Here's the drawing with two shaded views (mm, measured from the low corner). I have some questions. A direction names the side the tool comes from. Round coordinates to 2 decimals unless told otherwise and drop trailing zeros. Loops run counter-clockwise (first coordinate to the right, second up) from the corner with the lowest first, then second, coordinate; pieces in that order, holes last.
(1) Will these pins go through, and if not, where does the flat tip stop? pin 1 Ø5 at (x, y) = (19, 118) entering from -Z; pin 2 Ø10 at (x, z) = (13.5, 18.5) entering from -Y.
(2) Thinking about a two-plate mould opening in Z: for the marked faces 1, 2 and 3, which applies, released by +Z, released by -Z, zero draft, split by the parting line, or undercut?
(3) I want a section at B-B on y = 37. Write out the boundary of the cut face in (x, z).
(4) I want a section at C-C on x = 9. Write out the boundary of the cut face in (y, z) (1 decimal).
(5) I want a section at A-A on z = 20.25. Write out the boundary of the cut face in (x, y) (1 decimal), plus the area to 3 significant figures.
(6) If I drill on line 1 along X through (y, z) = (228, 19); line 2 along Z through (x, y) = (27.5, 200), over which ranges is the centre line in solid material (lowest first)?
(7) Which directions (+Z, -Z, +X, -X, +Y, -Y) give clear straight access to the entire face, cutting with the end or side of a thin tool? Please do the marked faces 4 and 5.
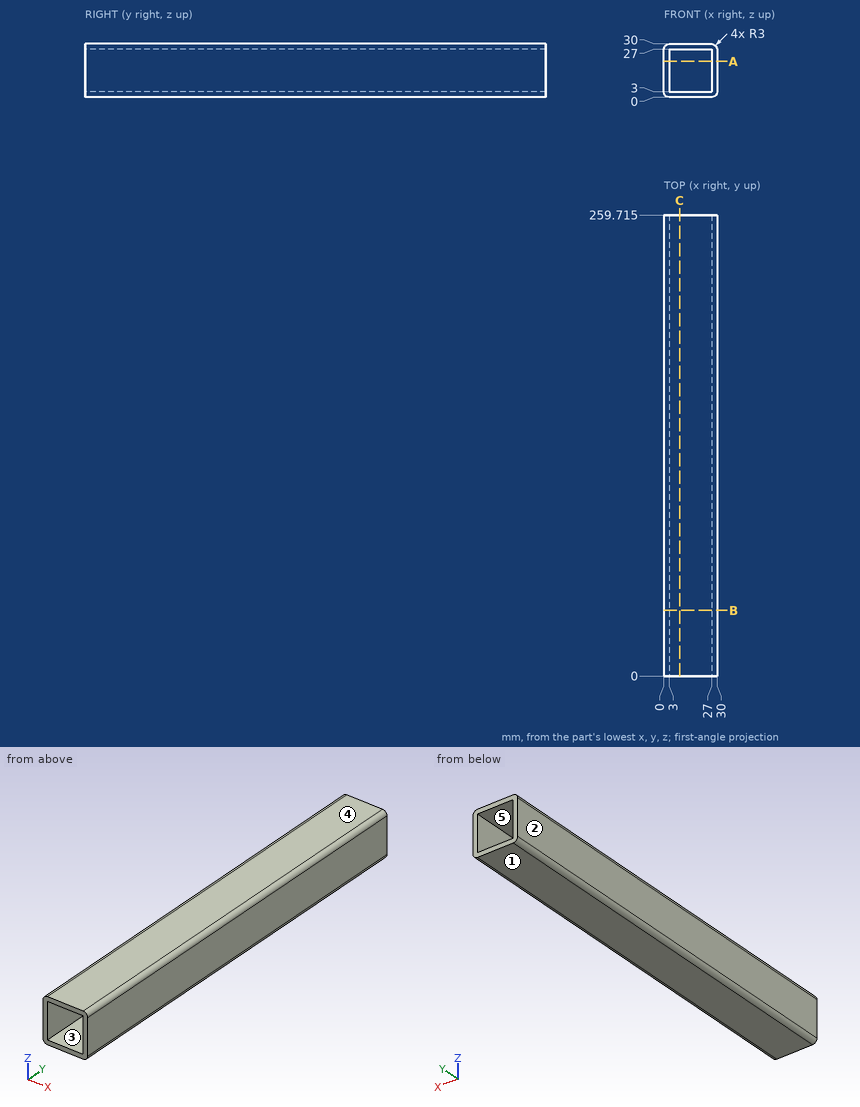
Filled sheet:
1. pin 1: stops at z = 0
1. pin 2: passes through
2. face 1: released by -Z
2. face 2: zero draft
2. face 3: undercut
3. outline: (0, 3) arc R3 ccw to (3, 0) - (27, 0) arc R3 ccw to (30, 3) - (30, 27) arc R3 ccw to (27, 30) - (3, 30) arc R3 ccw to (0, 27) - close; hole (3, 3) - (27, 3) - (27, 27) - (3, 27) - close
4. outline: (0, 0) - (259.7, 0) - (259.7, 3) - (0, 3) - close; (0, 27) - (259.7, 27) - (259.7, 30) - (0, 30) - close
5. outline: (0, 0) - (3, 0) - (3, 259.7) - (0, 259.7) - close; (27, 0) - (30, 0) - (30, 259.7) - (27, 259.7) - close
5. area: 1,560 mm2
6. line 1: x = 0 to 3, 27 to 30
6. line 2: z = 0.04 to 29.96
7. face 4: +Z, +X, -X, +Y, -Y
7. face 5: +Y, -Y
